Part model, mm, in its own coordinate system. Face numbers are marked on the shaded views. A direction names the side the tool comes from. Coordinates: 2 decimals unless noted, no trailing zeros. Loops run counter-clockwise (first coordinate to the right, second up) from the corner with the lowest first, then second, coordinate; pieces in that order, holes last. Notation, with made-up numbers: (75, -6) - (89, -6) arc R6 cw to (89, 3) - close; hole circle Ø2 at (-23, 16.5). An arc over 180 degrees is marked (long way). Answer as CSV lines item,"result".
from build123d import *

# Parameters (mm, degrees)
SKETCH1_W = 6
SKETCH1_H = 22.915


with BuildPart() as part:
    # Sketch1 → Revolve1 (revolve)
    with BuildSketch(Plane.XY, mode=Mode.PRIVATE) as revolve1_sk:
        with BuildLine():
            Line((-8.959217604, 38), (0, 19.085))
            Line((0, 19.085), (14.040782396, 19.085))
            Line((14.040782396, 19.085), (14.040782396, 42))
            Line((14.040782396, 42), (14.040782396, 45))
            ThreePointArc((14.040782396, 45), (13.16210274, 47.121320344), (11.040782396, 48))
            Line((11.040782396, 48), (-8.959217604, 48))
            Line((-8.959217604, 48), (-8.959217604, 38))
        make_face()
        with Locations((17.040782396, 30.5425)):
            Rectangle(SKETCH1_W, SKETCH1_H)
        Polygon((20.040782396, 42), (20.040782396, 19.085), (28.557506112, 19.085), (45.040782396, 19.085), (45.040782396, 40), (45.040782396, 48), (20.040782396, 48), align=None)
        with BuildLine():
            Line((57.520391198, 19.085), (57.520391198, 11.33900978))
            Line((57.520391198, 11.33900978), (95.040782396, 11.33900978))
            Line((95.040782396, 11.33900978), (95.040782396, 20))
            Line((95.040782396, 20), (65.313312444, 24.371686758))
            ThreePointArc((65.313312444, 24.371686758), (62.256779901, 26.050252773), (61.040782396, 29.318482435))
            Line((61.040782396, 29.318482435), (61.040782396, 38))
            ThreePointArc((61.040782396, 38), (60.454995958, 39.414213562), (59.040782396, 40))
            Line((59.040782396, 40), (54.186650367, 40))
            Line((54.186650367, 40), (45.040782396, 40))
            Line((45.040782396, 40), (45.040782396, 19.085))
            Line((45.040782396, 19.085), (57.520391198, 19.085))
        make_face()
        with BuildLine():
            Line((95.040782396, 11.33900978), (115.040782396, 11.33900978))
            Line((115.040782396, 11.33900978), (115.040782396, 17))
            ThreePointArc((115.040782396, 17), (114.16210274, 19.121320344), (112.040782396, 20))
            Line((112.040782396, 20), (95.040782396, 20))
            Line((95.040782396, 20), (95.040782396, 11.33900978))
        make_face()
    revolve(revolve1_sk.sketch.rotate(Axis((0, 0, 0), (1, 0, 0)), 90), axis=Axis((0, 0, 0), (1, 0, 0)))


solid = part.part
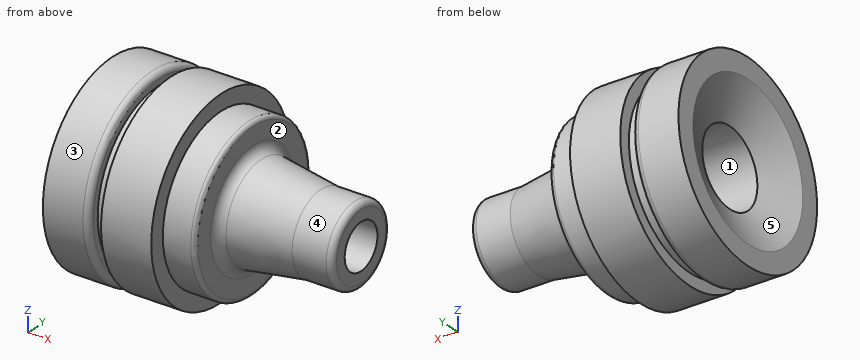
Q1. Saw through at B-B (x = 100.5). Give the cut face in (y, z), then the cut area to 3 significant figures.
Results:
outline,"circle Ø40 at (0, 0); hole circle Ø22.68 at (0, 0)"
area,"853 mm^2"
Q2. Saw through at A-A (x = 28.5). Give the cut face in (y, z) (3 decimals).
Results:
outline,"circle Ø96 at (0, 0); hole circle Ø38.17 at (0, 0)"
Q3. Wall check: L1, parallel to Y at x = 27.5, z = 0 (3 decimals); L2, parallel to X at y = 16, z = 1.5; L3, parallel to X at y = 17.5, z = -41. Give the ranges that are in metal, low to high.
Results:
L1,"y = -48 to -19.085, 19.085 to 48"
L2,"x = 57.52 to 115.04"
L3,"x = -8.96 to 14.04, 20.04 to 45.04"
Q4. Which spindle directions (+Z, -Z, +X, -X, +Y, -Y) get a long thin tool onto all of the face, cutting with end or side? Do the marked faces 4 and 5. Say none if no direction does.
Results:
face 4,"+X"
face 5,"-X"
Q5. Flat gauge pins, fed straight in: pin 1 (6 mm diameter, centred on x = 27.5, z = -23, fed in from +Y); pin 2 (5 mm diameter, centred on x = 44, y = 22, fed in from -Z); pin 3 (12 mm diameter, centred on x = 92.5, z = 15.5, fed in from +Y). Where does each tip first touch, or does it go through?
Results:
pin 1,"stops at y = 43.63"
pin 2,"stops at z = -43.86"
pin 3,"stops at y = 18.18"
Q6. Two-plate mould, pull along Y, no slides. Class the marked faces 1, 2 and 3: released by +Y, released by -Y, zero draft, split by the parting line, or undercut.
Results:
face 1,"undercut"
face 2,"zero draft"
face 3,"split by the parting line"
